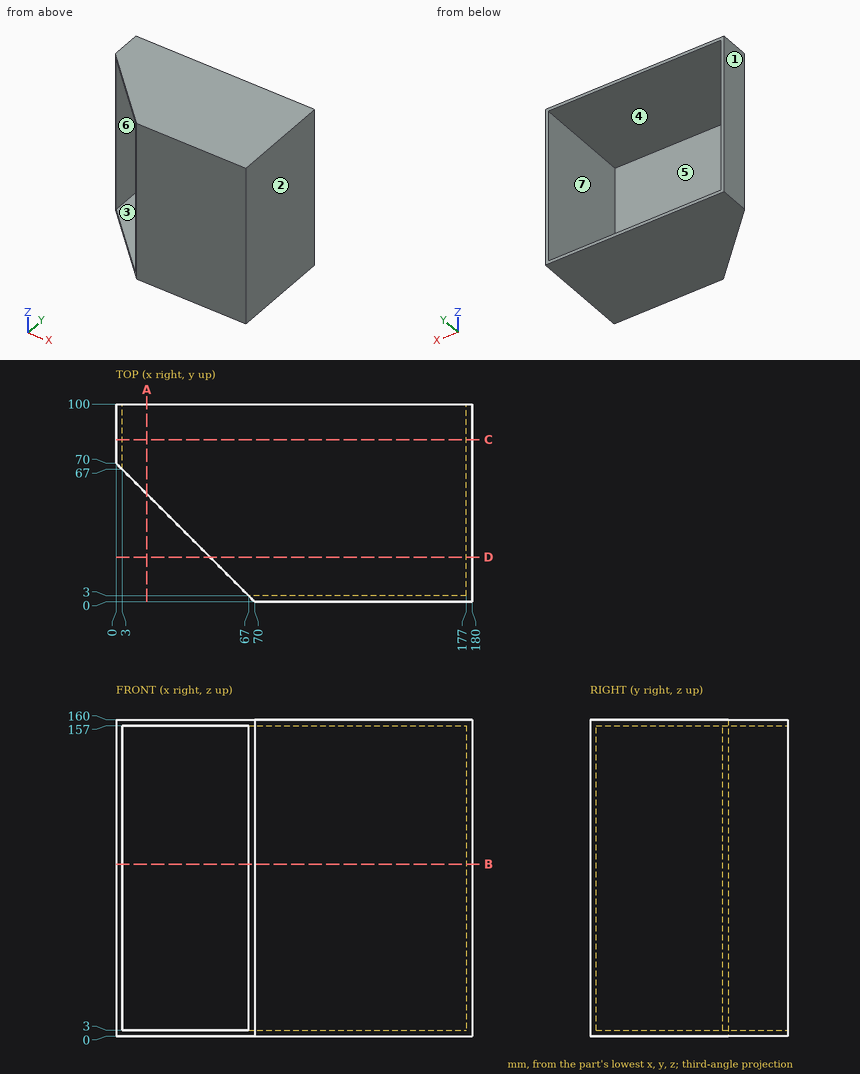
Drawing for the job (mm, zero at the part's lowest x, y, z). A direction names the side the tool comes from. Coordinates: 2 decimals unless noted, no trailing zeros. Order: outer loops, then holes, each group sorted by start corner. A loop starts at its lowest first (then second) coordinate and runs counter-clockwise, first axis right, second up. Notation, with made-up numbers: (-25.75, 58.25) -> (11.25, 58.25) arc R22 ccw to (11.25, 78.25) -> close; hole circle Ø3 at (87, 48.25). An arc over 180 degrees is marked (long way). Return JSON: item names as keys, results as strings.
Item 1: Slice it at A-A (x = 15.5). Write the cut outline in (y, z).
Model answer:
{"outline": "(54.5, 0) -> (100, 0) -> (100, 3) -> (54.5, 3) -> close; (54.5, 157) -> (100, 157) -> (100, 160) -> (54.5, 160) -> close"}
Item 2: Slice it at D-D (y = 22.5). Write the cut outline in (x, z).
Model answer:
{"outline": "(47.5, 0) -> (180, 0) -> (180, 160) -> (47.5, 160) -> (47.5, 157) -> (177, 157) -> (177, 3) -> (47.5, 3) -> close"}
Item 3: Wall check: line 1 along Z through (x, y) = (142, 5); line 2 along X through (y, z) = (94, 62); line 3 along X through (y, z) = (6.5, 26.5). Give the ranges that are in metal, low to high. Write a range as from..to.
Model answer:
{"line 1": "z = 0..3, 157..160", "line 2": "x = 0..3, 177..180", "line 3": "x = 177..180"}
Item 4: 3-axis set-ups, long thin cutter, end or side, ignore diameter. For the marked faces 5, 6 and 7: which of +Z, -Z, +X, -X, +Y, -Y reach the whole face in a straight line?
Model answer:
{"face 5": "-X, +Y", "face 6": "+Y, -Y", "face 7": "+Y"}
Item 5: Pin check, flat tips, straight feed: P1, Ø2, axis at y = 34.5, z = 111.5, coming from the -X side; P2, Ø10, axis at x = 94, z = 19.5, coming from the +Y side. Stop position of each tip, or through.
Model answer:
{"P1": "stops at x = 177", "P2": "stops at y = 3"}
Item 6: Mould opens along X. For the marked faces 1, 2, 3 and 4 say: pulls with the +X half, pulls with the -X half, needs draft (parallel to the pull), parting line crosses it, or undercut.
Model answer:
{"face 1": "pulls with the -X half", "face 2": "pulls with the +X half", "face 3": "undercut", "face 4": "undercut"}
Item 7: Slice it at C-C (y = 82). Write the cut outline in (x, z).
Model answer:
{"outline": "(0, 0) -> (180, 0) -> (180, 160) -> (0, 160) -> close; hole (3, 3) -> (177, 3) -> (177, 157) -> (3, 157) -> close"}
Item 8: Slice it at B-B (z = 87). Write the cut outline in (x, y).
Model answer:
{"outline": "(0, 70) -> (3, 67) -> (3, 100) -> (0, 100) -> close; (67, 3) -> (70, 0) -> (180, 0) -> (180, 100) -> (177, 100) -> (177, 3) -> close"}
